Read the model definition and answer for the solid it produces. Units are mm, in the model's axes. Face numbers are marked on the shaded views. Round coordinates to 2 decimals unless told otherwise and drop trailing zeros. Order: outer loops, then holes, each group sorted by start corner. A loop starts at its lowest first (then second) coordinate and runs counter-clockwise, first axis right, second up. Notation, with made-up numbers: (-15.75, 53.25) -> (21.25, 53.25) arc R23 ccw to (21.25, 69.25) -> close; hole circle Ø2 at (25, 56.5). An arc over 180 degrees is marked (long way). Use a Markdown table: item, result. Add a question column.
1. Consider L1, parallel to X at y = -1.5, z = 2.4; L2, parallel to X at y = -2, z = 2.05; L3, parallel to Y at x = 0, z = 1.75. Determine where each line is inside the solid, lowest interval first. Write a range as [from, to].
2. Section D-D, the plane y = -13 is taken. Give the vertices of the cut face in (x, z), then the cut area to 3 significant figures.
3. The mould has two halves that part along Y. Classify the marked faces 1, 2, 3 and 4: +Y half, -Y half, draft (parallel to the pull), parting line (faces both ways), or undercut.
4. Section C-C, the plane y = 0 is taken. Give the number of separate pieces and of enclosed holes in the cut face, then the cut area to 3 significant figures.
5. Section B-B, the plane z = 0.5 is taken. Give the vertices of the cut face in (x, y) (3 decimals).
6. Section A-A, the plane x = 0 is taken. Give the vertices of the cut face in (y, z).
```python
from build123d import *

# Parameters (mm, degrees)
SKETCH1_R           = 20.5
BOSS_EXTRUDE1_DEPTH = 2.9
SKETCH2_R           = 1.275
CUT_EXTRUDE1_DEPTH  = 30.136060132
CHAMFER1_SIZE       = 1.6
CHAMFER1_SIZE2      = 1.390858781
SKETCH3_R           = 5.5
CUT_EXTRUDE2_DEPTH  = 30.136060132


with BuildPart() as part:
    # Sketch1 → Boss-Extrude1 (new body)
    with BuildSketch(Plane.XY):
        Circle(SKETCH1_R)
    extrude(amount=BOSS_EXTRUDE1_DEPTH)

    # Sketch2 → Cut-Extrude1 (cut, through all)
    with BuildSketch(Plane.XY.offset(2.9)):
        with Locations((-8.971859678, -0.711149714)):
            Circle(SKETCH2_R)
        with Locations((5.101803557, -7.414283544)):
            Circle(SKETCH2_R)
        with Locations((3.870056121, 8.125433257)):
            Circle(SKETCH2_R)
    extrude(amount=-CUT_EXTRUDE1_DEPTH, mode=Mode.SUBTRACT)

    # Chamfer1
    chamfer1_edges = [part.edges().sort_by_distance(p)[0] for p in [
        (3.826803557, -7.414283544, 2.9),
        (2.595056121, 8.125433257, 2.9),
        (-10.246859678, -0.711149714, 2.9),
    ]]
    chamfer1_side = [part.faces().sort_by_distance(p)[0] for p in [
        (0, 0, 2.9),
    ]]
    chamfer(chamfer1_edges, length=CHAMFER1_SIZE, length2=CHAMFER1_SIZE2, reference=chamfer1_side[0])

    # Sketch3 → Cut-Extrude2 (cut, through all)
    with BuildSketch(Plane.XY.offset(2.9)):
        Circle(SKETCH3_R)
    extrude(amount=-CUT_EXTRUDE2_DEPTH, mode=Mode.SUBTRACT)


solid = part.part
```
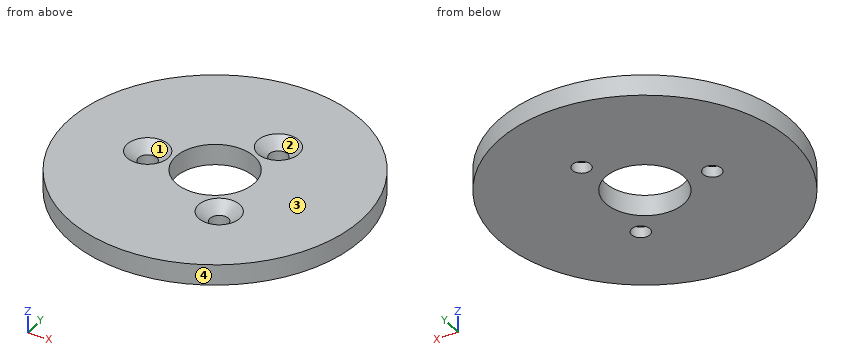
Verdict:
| question | item | result |
|---|---|---|
| 1 | L1 | x = [-20.45, -11.13], [-6.81, -5.29], [5.29, 20.45] |
| 1 | L2 | x = [-20.4, -10.36], [-7.58, -5.12], [5.12, 20.4] |
| 1 | L3 | y = [-20.5, -5.5], [5.5, 20.5] |
| 2 | outline | (-15.85, 0) -> (15.85, 0) -> (15.85, 2.9) -> (-15.85, 2.9) -> close |
| 2 | area | 91.9 mm2 |
| 3 | face 1 | undercut |
| 3 | face 2 | undercut |
| 3 | face 3 | draft |
| 3 | face 4 | parting line |
| 4 | separate pieces | 3 |
| 4 | enclosed holes | 0 |
| 4 | area | 78.4 mm2 |
| 5 | outline | circle Ø41 at (0, 0); hole circle Ø2.55 at (-8.972, -0.711); hole circle Ø11 at (0, 0); hole circle Ø2.55 at (3.87, 8.125); hole circle Ø2.55 at (5.102, -7.414) |
| 6 | outline | (-20.5, 0) -> (-5.5, 0) -> (-5.5, 2.9) -> (-20.5, 2.9) -> close; (5.5, 0) -> (20.5, 0) -> (20.5, 2.9) -> (5.5, 2.9) -> close |
